Could you check a few things on this model? Use its own coordinates, in mm. A direction names the side the tool comes from. Coordinates: 2 decimals unless noted, no trailing zeros. Write each loop counter-clockwise with the first axis right and the second up, starting at its lowest first coordinate (ties: lowest second). Pieces come first, ordered by that corner, then holes. Notation, with made-up numbers: M 25,49 L 79,49 A10 cw 79,57 Z; hole C 15.5,27 d4. An arc over 180 degrees is marked long. Write item = value, one per line.
```python
from build123d import *

# Parameters (mm, degrees)
F1_DEPTH = 63.5
F0_W     = 19.151572957
F0_H     = 19.05
F2_DEPTH = 38.1
F3_DEPTH = 12.7


with BuildPart() as f1:
    # F0 (on Front) → F1 (new body, symmetric)
    with BuildSketch(Plane.XZ):
        Polygon((19.05, 15.875), (-38.1, 15.875), (-38.1, -15.875), (38.1, -15.875), (38.1, 15.875), align=None)
    extrude(amount=F1_DEPTH, both=True)

    # F0 (on Front) → F2 (join, symmetric)
    with BuildSketch(Plane.XZ):
        with BuildLine():
            Line((19.05, 32.0585994233), (19.05, 15.875))
            Line((19.05, 15.875), (38.1, 15.875))
            Line((38.1, 15.875), (38.1, 32.0585994233))
            ThreePointArc((38.1, 32.0585994233), (43.3076414305, 44.6309579928), (55.88, 49.8385994233))
            Line((55.88, 49.8385994233), (76.2, 49.8385994233))
            Line((76.2, 49.8385994233), (76.2, 68.8885994233))
            Line((76.2, 68.8885994233), (55.88, 68.8885994233))
            ThreePointArc((55.88, 68.8885994233), (29.8372572489, 58.1013421744), (19.05, 32.0585994233))
        make_face()
        with Locations((85.7757864785, 59.3635994233)):
            Rectangle(F0_W, F0_H)
    extrude(amount=F2_DEPTH, both=True)

    # F0 (on Front) → F3 (join, symmetric)
    with BuildSketch(Plane.XZ):
        with BuildLine():
            add(Edge.make_bspline(
                [(-38.1, 15.875), (-36.8803367019, 43.9477860928), (14.5305916667, 69.8257684708), (55.88, 68.8885994233)],
                knots=[0, 0, 0, 0, 107.9012609927, 107.9012609927, 107.9012609927, 107.9012609927], degree=3))
            Line((-38.1, 15.875), (19.05, 15.875))
            Line((19.05, 15.875), (19.05, 32.0585994233))
            ThreePointArc((19.05, 32.0585994233), (29.8372572489, 58.1013421744), (55.88, 68.8885994233))
        make_face()
    extrude(amount=F3_DEPTH, both=True)

    # F0 (on Front) → F4 (revolve)
    with BuildSketch(Plane.XZ):
        Polygon((95.351572957, 93.3624118266), (95.351572957, 68.8885994233), (95.351572957, 49.8385994233), (95.351572957, 29.8624118266), (127, 29.8624118266), (127, 93.3624118266), align=None)
    revolve(axis=Axis((95.351572957, 0, 61.6124118266), (0, 0, 1)))


solid = f1.part
```
Item 1: Imagine slicing it at A-A (z = 80). Write out the boundary of the cut face in (x, y), and give its area (3 significant figures).
Numbers:
outline = C 95.35,0 d63.3
area = 3,150 mm²
Item 2: Imagine slicing it at B-B (y = 26). Write out the boundary of the cut face in (x, z) (3 decimals), and give its area (3 significant figures).
Numbers:
outline = M -38.1,-15.875 L 38.1,-15.875 L 38.1,32.059 A17.78 cw 55.88,49.839 L 77.307,49.839 L 77.307,29.862 L 113.397,29.862 L 113.397,93.362 L 77.307,93.362 L 77.307,68.889 L 55.88,68.889 A36.83 ccw 19.05,32.059 L 19.05,15.875 L -38.1,15.875 Z
area = 6,240 mm²
Item 3: For faces 5 (the face through (95.352, 35, 59)), 6 (the face through (-1, -12.7, 37)), 7 (the face through (48, -38.1, 49)), 8 (the face through (96, 0, 29.862)), which set-ups out of +Z, -Z, +X, -X, +Y, -Y let a thin tool reach every point of the face, with its end or its side?
Numbers:
face_5 = +Z, -Z, +X, +Y
face_6 = +Z, -X, -Y
face_7 = +Z, +X, -X, -Y
face_8 = -Z, +X, +Y, -Y
Item 4: If we mould it in two halves opening along X, with no side actions, what happens to faces 1 (the face through (30.13, 25.22, 58.39)), 2 (the face through (62, -1, 49.839)), 3 (the face through (-1, -1, -15.875)), 4 (the face through (43.17, -0.53, 44.49))? For each: pulls with the +X half, pulls with the -X half, needs draft (parallel to the pull), parting line crosses it, or undercut.
Numbers:
face_1 = pulls with the -X half
face_2 = undercut
face_3 = needs draft
face_4 = undercut
Item 5: Imagine slicing it at D-D (z = -1). Write out the boundary of the cut face in (x, y).
Numbers:
outline = M -38.1,-63.5 L 38.1,-63.5 L 38.1,63.5 L -38.1,63.5 Z
Item 6: Imagine slicing it at C-C (y = -46). Write out the boundary of the cut face in (x, z) (3 decimals), and give its area (3 significant figures).
Numbers:
outline = M -38.1,-15.875 L 38.1,-15.875 L 38.1,15.875 L -38.1,15.875 Z
area = 2,420 mm²
Item 7: I'm going to push flat-ended pins straight in: P1, Ø16, axis at x = 39.5, z = 35, coming from the -Y side; P2, Ø7, axis at y = -36.5, z = 62.5, coming from the +X side; P3, Ø8, axis at y = -31, z = 24.5, coming from the -X side. Where does each tip first touch, or does it pass through?
Numbers:
P1 = -38.1
P2 = 95.35
P3 = 19.05
Item 8: If I drill on line 1 along X through (y, z) = (20.5, 28); line 2 along Z through (x, y) = (97, 24); line 3 along Z through (x, y) = (58, 13), over which ranges is the centre line in solid material (lowest first)?
Numbers:
line_1 = 19.05 to 38.1
line_2 = 29.86 to 93.36
line_3 = 49.84 to 68.89
